Build history of the part. All positions in model axes, mm. Round coordinates to 2 decimals unless told otherwise and drop trailing zeros. Loops run counter-clockwise (first coordinate to the right, second up) from the corner with the lowest first, then second, coordinate; pieces in that order, holes last. Notation, with made-up numbers: (32, 84) -> (38, 84) arc R15 cw to (38, 106) -> close; hole circle Ø6 at (34, -4). An arc over 180 degrees is marked (long way). Put each result on its own line as item: value. Start each with the question number.
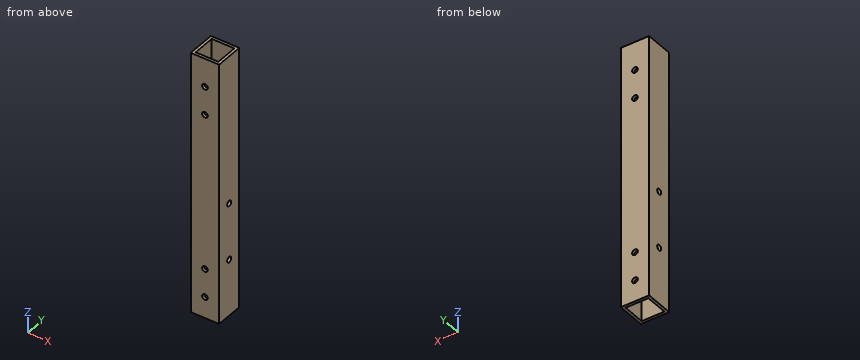
```python
from build123d import *

# Parameters (mm, degrees)
SKETCH_1_W          = 20
SKETCH_1_H          = 20
SKETCH_1_W_2        = 16
SKETCH_1_H_2        = 16
EXTRUDE_1_DEPTH     = 185
SKETCH_2_R          = 2
CUT_EXTRUDE_1_DEPTH = 187.346451536
SKETCH_3_R          = 2
CUT_EXTRUDE_2_DEPTH = 187.346451536


with BuildPart() as part:
    # 草图1 → 凸台-拉伸1 (new body)
    with BuildSketch(Plane.XY):
        Rectangle(SKETCH_1_W, SKETCH_1_H)
        Rectangle(SKETCH_1_W_2, SKETCH_1_H_2, mode=Mode.SUBTRACT)
    extrude(amount=EXTRUDE_1_DEPTH)

    # 草图2 → 切除-拉伸1 (cut, through all)
    with BuildSketch(Plane(origin=(0, 10, 0), x_dir=(1, 0, 0), z_dir=(0, 1, 0))):
        with Locations(Location((0, -15, 0), (0, 0, 180))):
            Circle(SKETCH_2_R)
        with Locations(Location((0, -35, 0), (0, 0, 180))):
            Circle(SKETCH_2_R)
        with Locations(Location((0, -165, 0), (0, 0, 180))):
            Circle(SKETCH_2_R)
        with Locations(Location((0, -145, 0), (0, 0, 180))):
            Circle(SKETCH_2_R)
    extrude(amount=-CUT_EXTRUDE_1_DEPTH, mode=Mode.SUBTRACT)

    # 草图3 → 切除-拉伸2 (cut, through all)
    with BuildSketch(Plane.ZY.offset(10)):
        with Locations((40, 0)):
            Circle(SKETCH_3_R)
        with Locations((80, 0)):
            Circle(SKETCH_3_R)
    extrude(amount=-CUT_EXTRUDE_2_DEPTH, mode=Mode.SUBTRACT)


solid = part.part
```
Item 1: Cut at A-A on y = -5. Write the cut outline in (x, z), then the cut area to 3 significant figures.
Item 2: Drop a flat-ended pin along its axis: pin 1 (3 mm diameter, centred on x = 5.5, y = -7.5, fed in from -Z). Give the stop position or say it passes through.
Item 3: Wall check: line 1 (Z direction, x = 0, y = 9.1); line 2 (Y direction, x = -0.75, z = 160). Give the ranges that are in metal, low to high. Write a range as from..to.
Item 4: Cut at C-C on z = 15. Write the cut outline in (x, y), then the cut area to 3 significant figures.
Ans:
1. outline: (-10, 0) -> (-8, 0) -> (-8, 185) -> (-10, 185) -> close; (8, 0) -> (10, 0) -> (10, 185) -> (8, 185) -> close
1. area: 740 mm2
2. pin 1: stops at z = 0
3. line 1: z = 0..13, 17..33, 37..143, 147..163, 167..185
3. line 2: y = -10..-8, 8..10
4. outline: (-10, -10) -> (-2, -10) -> (-2, -8) -> (-8, -8) -> (-8, 8) -> (-2, 8) -> (-2, 10) -> (-10, 10) -> close; (2, -10) -> (10, -10) -> (10, 10) -> (2, 10) -> (2, 8) -> (8, 8) -> (8, -8) -> (2, -8) -> close
4. area: 128 mm2
